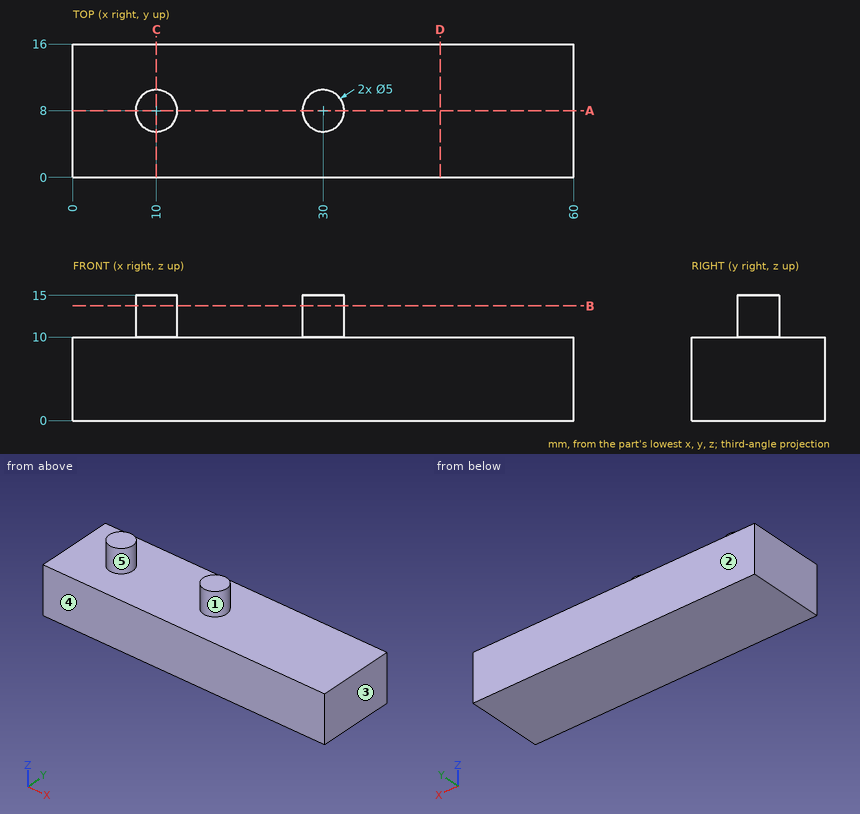
The drawing under review shows one solid part. Ordinate dimensions are in mm from its lowest x, y, z. A direction names the side the tool comes from. Round coordinates to 2 decimals unless told otherwise and drop trailing zeros. Write each loop counter-clockwise with the first axis right and the second up, starting at its lowest first coordinate (ties: lowest second). Pieces come first, ordered by that corner, then holes. Notation, with made-up numbers: (22.25, -23) - (35.25, -23) arc R22 ccw to (35.25, -10) - close; hole circle Ø1 at (19, -37.75). An arc over 180 degrees is marked (long way). Use a Markdown table: item, result. Add a question column.
1. Wall thickness on probe 1 along X at (y, z) = (7.75, 11.25); probe 2 along Z at (x, y) = (7.5, 10); probe 3 along X at (y, z) = (7.5, 11.5): over which ranges is each line inside the solid? List them lowest first.
2. For the marked faces 1 and 2, list the 3-axis set-ups (+Z, -Z, +X, -X, +Y, -Y) from which the entire face can be reached by the end or side of a thin tool; tool diameter is ignored.
3. We need section C-C (x = 10). State the section outline as (y, z) points.
4. We need section A-A (y = 8). State the section outline as (x, z) points.
5. We need section D-D (x = 44). State the section outline as (y, z) points, then the cut area to 3 significant figures.
6. Mouldability with a two-part tool opening along X and no side actions: class the marked faces 3, 4 and 5 as +X half, -X half, draft (parallel to the pull), parting line (faces both ways), or undercut.
7. We need section B-B (z = 13.75). State the section outline as (x, y) points, then the cut area to 3 significant figures.
Output:
| question | item | result |
|---|---|---|
| 1 | probe 1 | x = 7.51 to 12.49, 27.51 to 32.49 |
| 1 | probe 2 | z = 0 to 10 |
| 1 | probe 3 | x = 7.55 to 12.45, 27.55 to 32.45 |
| 2 | face 1 | +Z |
| 2 | face 2 | +Z, -Z, +X, -X, +Y |
| 3 | outline | (0, 0) - (16, 0) - (16, 10) - (10.5, 10) - (10.5, 15) - (5.5, 15) - (5.5, 10) - (0, 10) - close |
| 4 | outline | (0, 0) - (60, 0) - (60, 10) - (32.5, 10) - (32.5, 15) - (27.5, 15) - (27.5, 10) - (12.5, 10) - (12.5, 15) - (7.5, 15) - (7.5, 10) - (0, 10) - close |
| 5 | outline | (0, 0) - (16, 0) - (16, 10) - (0, 10) - close |
| 5 | area | 160 mm2 |
| 6 | face 3 | +X half |
| 6 | face 4 | draft |
| 6 | face 5 | undercut |
| 7 | outline | circle Ø5 at (10, 8); circle Ø5 at (30, 8) |
| 7 | area | 39.3 mm2 |
